Check sheet for the modelled part. Datum: model origin and axes. Units: mm. A direction names the side the tool comes from. Give positions to 0.01 mm unless a question says otherwise; leave off trailing zeros. Write each loop counter-clockwise with the first axis right and the second up, starting at its lowest first coordinate (ties: lowest second). Pieces come first, ordered by that corner, then holes. Notation, with made-up numbers: (23.5, 44) -> (50.5, 44) arc R10 ccw to (50.5, 49) -> close; hole circle Ø1 at (30.25, -18.5). An arc over 180 degrees is marked (long way). Return JSON: item names as keys, results as strings.
from build123d import *

# Parameters (mm, degrees)
F0_W     = 11
F0_H     = 11
F1_DEPTH = 7
F2_SIZE  = 0.5


with BuildPart() as f1:
    # F0 (on Top) → F1 (new body)
    with BuildSketch(Plane.XY):
        Rectangle(F0_W, F0_H)
        with BuildLine():
            ThreePointArc((1.254631, 1.22), (0, -1.75), (-1.254631, 1.22))
            Line((-1.254631, 1.22), (1.254631, 1.22))
        make_face(mode=Mode.SUBTRACT)
    extrude(amount=F1_DEPTH)

    # F2
    f2_edges = [f1.edges().sort_by_distance(p)[0] for p in [
        (5.5, 0, 0),
        (0, 5.5, 0),
        (-5.5, 0, 0),
        (0, -5.5, 0),
        (0, 1.22, 0),
        (0, -1.75, 0),
    ]]
    chamfer(f2_edges, length=F2_SIZE)


solid = f1.part
(1) Thickness scan on L1, parallel to X at y = 0, z = 2; L2, parallel to Y at x = 0, z = 4.5; L3, parallel to Y at x = 1, z = 6.75. Record the ranges inside material, lowest first.
Reply:
{"L1": "-5.5 to -1.75, 1.75 to 5.5", "L2": "-5.5 to -1.75, 1.22 to 5.5", "L3": "-5.5 to -1.44, 1.22 to 5.5"}
(2) Release check for a two-part mould opening along Y. For faces 1 (the flat face through (-5.5, 0, 4)), 2 (the cylindrical face through (0.06, -1.75, 3.7)), 3 (the flat face through (0, -5.5, 4)) record: pulls with the +Y half, pulls with the -Y half, needs draft (parallel to the pull), parting line crosses it, or undercut.
Reply:
{"face 1": "needs draft", "face 2": "undercut", "face 3": "pulls with the -Y half"}
(3) Depth check by flat-ended pin: pin 1 Ø4 at (x, y) = (0, 0) entering from +Z. Enter the tip coordinate at first touch or a pass-through.
Reply:
{"pin 1": "z = 7"}
(4) Cross-section at C-C on z = 4.5. Enter the section's corners in (x, y), then the cut area to 3 significant figures.
Reply:
{"outline": "(-5.5, -5.5) -> (5.5, -5.5) -> (5.5, 5.5) -> (-5.5, 5.5) -> close; hole (-1.25, 1.22) arc R1.75 ccw (long way) to (1.25, 1.22) -> close", "area": "112 mm^2"}
(5) Set-up check for faces 4 (the flat face through (0, 1.22, 4)), 5 (the conical face through (0.06, -1.89, 0.36)): record each of +Z, -Z, +X, -X, +Y, -Y from which the full face is reachable in a straight line by a thin tool's end or side.
Reply:
{"face 4": "+Z, -Z", "face 5": "-Z"}
(6) Cross-section at A-A on x = 0. Enter the section's corners in (y, z), then the cut area to 3 significant figures.
Reply:
{"outline": "(-5.5, 0.5) -> (-5, 0) -> (-2.25, 0) -> (-1.75, 0.5) -> (-1.75, 7) -> (-5.5, 7) -> close; (1.22, 0.5) -> (1.72, 0) -> (5, 0) -> (5.5, 0.5) -> (5.5, 7) -> (1.22, 7) -> close", "area": "55.7 mm^2"}
(7) Cross-section at B-B on y = 0. Enter the section's corners in (x, z), then the cut area to 3 significant figures.
Reply:
{"outline": "(-5.5, 0.5) -> (-5, 0) -> (-2.25, 0) -> (-1.75, 0.5) -> (-1.75, 7) -> (-5.5, 7) -> close; (1.75, 0.5) -> (2.25, 0) -> (5, 0) -> (5.5, 0.5) -> (5.5, 7) -> (1.75, 7) -> close", "area": "52.0 mm^2"}
